Could you check a few things on this model? Use its own coordinates, in mm. Face numbers are marked on the shaded views. A direction names the side the tool comes from. Give positions to 0.01 mm unless a question says otherwise; leave off trailing zeros. Loops run counter-clockwise (first coordinate to the right, second up) from the corner with the lowest first, then second, coordinate; pieces in that order, holes last.
1. Thinking about a two-plate mould opening in Y: for the marked faces 3, 4 and 5, which applies, +Y half, -Y half, draft (parallel to the pull), parting line (faces both ways), or undercut?
2. For P1, Ø3, axis at y = 56, z = -381, coming from the -X side; P2, Ø5, axis at x = -131, y = 59, coming from the -Z side; P3, Ø12, axis at y = 32.5, z = -413, coming from the +X side, each with a flat end and sliding along its axis, tell me the tip position at first contact or that it passes through.
3. Imagine slicing it at B-B (x = -112). List the corners of the cut face in (y, z) for me, plus the area to 3 significant figures.
4. Imagine slicing it at A-A (z = -339). List the corners of the cut face in (x, y) for me, plus the area to 3 significant figures.
5. For the marked faces 1 and 2, which set-ups out of +Z, -Z, +X, -X, +Y, -Y let a thin tool reach every point of the face, with its end or its side?
6. I need wall thicknesses on line 1 along X through (y, z) = (107.5, -265); line 2 along X through (y, z) = (31, -170.5); line 3 along Y through (x, z) = (-447.5, -844). Which ranges of each line are inside material? Lowest first, please.
Autodesk Inventor part; units mm, degrees
ref_plane "YZ Plane" through (0, 0, 0) normal (1, 0, 0) x (0, 1, 0)
ref_plane "XZ Plane" through (0, 0, 0) normal (0, 1, 0) x (-1, 0, 0)
ref_plane "XY Plane" through (0, 0, 0) normal (0, 0, 1) x (1, 0, 0)
sketch "Эскиз1" plane through (0, 0, 0) normal (0, 0, 1) x (1, 0, 0)
  line L0 (0, 0) -> (0, 130)
  line L1 (0, 0) -> (130, 0)
  line L2 (130, 0) -> (0, 130)
  dimension "d0" = 130
  dimension "d1" = 130
sketch "Эскиз2" plane through (0, 0, 0) normal (0, 1, 0) x (-1, 0, 0)
  point P0 (0, 0)
sketch "Эскиз3" plane through (0, 0, 0) normal (0, 1, 0) x (-1, 0, 0)
  point P0 (0, 0)
sketch "Эскиз4" plane through (0, 0, 0) normal (0, 0, 1) x (1, 0, 0)
  line L0 (0, 0) -> (10, 0)
  line L1 (10, 10) -> (10, 110)
  line L2 (10, 10) -> (110, 10)
  line L3 (110, 10) -> (10, 110)
  dimension "d3" = 10
  dimension "d4" = 100
  dimension "d5" = 100
sketch "Эскиз5" plane through (0, 0, 0) normal (0, 1, 0) x (-1, 0, 0)
  line L0 (0, 0) -> (0, -388.8774)
  line L1 (82.4884, -574.4573) -> (238.5702, -715.3428)
  line L2 (406.0818, -779.7629) -> (809.939, -779.7629)
  arc A0 (0, -388.8774) -> (82.4884, -574.4573) centre (250, -388.8774) ccw
  arc A1 (238.5702, -715.3428) -> (406.0818, -779.7629) centre (406.0818, -529.7629) ccw
  point P0 (0, -500)
  point P1 (309.939, -779.7629)
  dimension "d6" = 500
  dimension "d7" = 500
  dimension "d8" = 250
sketch "Эскиз6" plane through (0, 0, 0) normal (0, 1, 0) x (-1, 0, 0)
  point P0 (0, 0)
sketch "Эскиз7" plane through (0, 0, 0) normal (0, 0, 1) x (1, 0, 0)
  point P0 (0, 0)
sweep "Сдвиг1" add profiles "Эскиз1" path "Эскиз5"
sketch3d "3D эскиз1"
  line L0 (0, 0, 0) -> (0, 0, -388.8774)
  arc A0 (0, 0, -388.8774) -> (-82.4884, 0, -574.4573) centre (-250, 0, -388.8774) ccw
  line L1 (-82.4884, 0, -574.4573) -> (-238.5702, 0, -715.3428)
  arc A1 (-238.5702, 0, -715.3428) -> (-406.0818, 0, -779.7629) centre (-406.0818, 0, -529.7629) ccw
  line L2 (-406.0818, 0, -779.7629) -> (-809.939, 0, -779.7629)
sweep "Сдвиг2" cut profiles "Эскиз4" path "3D эскиз1"
properties part number "lab_4_4"
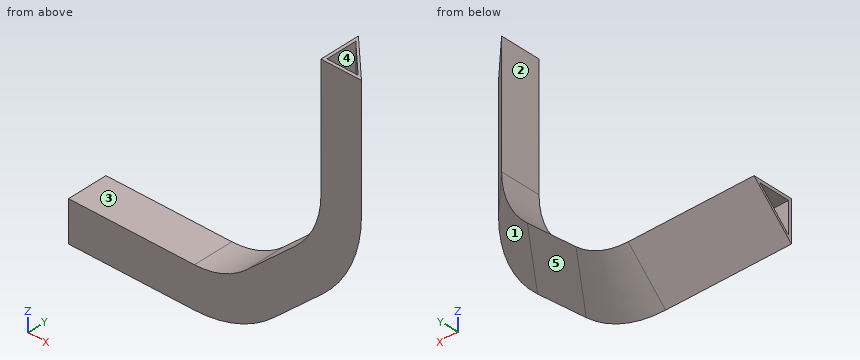
Derived:
1. face 3: draft
1. face 4: undercut
1. face 5: +Y half
2. P1: stops at x = 0
2. P2: stops at z = -717.95
2. P3: stops at x = 102.69
3. outline: (0, -776.22) - (130, -601.1) - (0, -601.1) - close; hole (10, -749.28) - (110, -614.57) - (10, -614.57) - close
3. area: 4,650 mm2
4. outline: (0, 0) - (130, 0) - (0, 130) - close; hole (10, 10) - (110, 10) - (10, 110) - close
4. area: 3,450 mm2
5. face 1: -Z, +X, +Y
5. face 2: +Z, -X, +Y, -Y
6. line 1: x = 0 to 10, 12.5 to 22.5
6. line 2: x = 0 to 10, 89 to 99
6. line 3: y = 0 to 10, 55.76 to 65.76
